The model under review builds one solid part; all positions refer to its coordinate system, in mm. A direction names the side the tool comes from. Round coordinates to 2 decimals unless told otherwise and drop trailing zeros. Loops run counter-clockwise (first coordinate to the right, second up) from the corner with the lowest first, then second, coordinate; pieces in that order, holes last. Notation, with made-up numbers: (49.25, 20.25) -> (65.25, 20.25) arc R26 ccw to (65.25, 37.25) -> close; hole circle Ø4 at (-1, -12.75). An arc over 180 degrees is marked (long way). Use a Markdown table: item, result. Add a question column.
1) For faces 5 (the flat face through (-29, 12, 0)), 6 (the flat face through (-73, -33.454, 1)), 7 (the flat face through (-65, 17.146, 1)), 8 (the flat face through (9.821, 11, 1)), 9 (the cylindrical face through (-4.345, 10.69, 0.986)), list the 3-axis set-ups (+Z, -Z, +X, -X, +Y, -Y) from which the entire face can be reached by the end or side of a thin tool; tool diameter is ignored.
2) Consider section B-B on y = 13.5. Give the boundary of the cut face in (x, z), plus the area to 3 significant figures.
3) Mouldability with a two-part tool opening along Y and no side actions: class faces 1 (the flat face through (0.818, -17.776, 0.986)), 2 (the flat face through (6.821, 16, 1)), 3 (the flat face through (2, 21.146, 1)), 4 (the flat face through (11.321, -30, 1)) as released by +Y, released by -Y, zero draft, split by the parting line, or undercut.
4) Consider section A-A on x = -11.5. Give the boundary of the cut face in (y, z).
5) Wall thickness on probe 1 along Y at (x, z) = (-65.5, 0.2); probe 2 along X at (y, z) = (15.5, 1.3); probe 3 along Y at (x, z) = (-35.5, 1.35): over which ranges is each line inside the solid? List them lowest first.
6) Insertion check: pin 1 (1 mm diameter, centred on x = 8.5, z = 1.5, fed in from -Y); pin 2 (0.8 mm diameter, centred on x = 10, z = 1, fed in from +Y); pin 3 (0.6 mm diameter, centred on y = 20, z = 1, fed in from +X). Each pin has a flat end and moves straight along its axis. Give the tip position at first contact, or say it passes through.
7) Consider section C-C on y = -3.5. Give the boundary of the cut face in (x, z), plus the area to 3 significant figures.
from build123d import *

# Parameters (mm, degrees)
EXTRUDE_1_DEPTH = 2


with BuildPart() as part:
    # 草图1 → 凸台-拉伸1 (new body)
    with BuildSketch(Plane.XY):
        Polygon((-63.278571429, -35.454285714), (-63.278571429, -33.454285714), (-65.778571429, -33.454285714), (-65.778571429, -30.954285714), (-64.278571429, -30.954285714), (-64.278571429, -28.354285714), (-65.778571429, -28.354285714), (-65.778571429, -25.354285714), (-68.778571429, -25.354285714), (-68.778571429, -28.354285714), (-70.278571429, -28.354285714), (-70.278571429, -30.954285714), (-68.778571429, -30.954285714), (-68.778571429, -33.454285714), (-77.278571429, -33.454285714), (-77.278571429, 17.145714286), (-68.778571429, 17.145714286), (-68.778571429, 14.645714286), (-70.278571429, 14.645714286), (-70.278571429, 12.045714286), (-68.778571429, 12.045714286), (-68.778571429, 9.045714286), (-65.778571429, 9.045714286), (-65.778571429, 12.045714286), (-64.278571429, 12.045714286), (-64.278571429, 14.645714286), (-65.778571429, 14.645714286), (-65.778571429, 17.145714286), (-63.278571429, 17.145714286), (-63.278571429, 21.145714286), (-59.478571429, 21.145714286), (-59.478571429, 17.145714286), (0.521428571, 17.145714286), (0.521428571, 21.145714286), (4.321428571, 21.145714286), (4.321428571, 17.145714286), (6.821428571, 17.145714286), (6.821428571, 14.645714286), (5.321428571, 14.645714286), (5.321428571, 12.045714286), (6.821428571, 12.045714286), (6.821428571, 9.045714286), (9.821428571, 9.045714286), (9.821428571, 12.045714286), (11.321428571, 12.045714286), (11.321428571, 14.645714286), (9.821428571, 14.645714286), (9.821428571, 17.145714286), (17.321428571, 17.145714286), (17.321428571, -33.454285714), (9.821428571, -33.454285714), (9.821428571, -30.954285714), (11.321428571, -30.954285714), (11.321428571, -28.354285714), (9.821428571, -28.354285714), (9.821428571, -25.354285714), (6.821428571, -25.354285714), (6.821428571, -28.354285714), (5.321428571, -28.354285714), (5.321428571, -30.954285714), (6.821428571, -30.954285714), (6.821428571, -33.454285714), (4.321428571, -33.454285714), (4.321428571, -35.454285714), (0.521428571, -35.454285714), (0.521428571, -33.454285714), (-59.478571429, -33.454285714), (-59.478571429, -35.454285714), align=None)
        with BuildLine():
            Line((-5.934446775, 11.145714286), (-52.852891654, 11.145714286))
            ThreePointArc((-52.852891654, 11.145714286), (-54.499158877, 10.653662497), (-55.605393612, 9.338917105))
            Line((-55.605393612, 9.338917105), (-62.671403465, -6.961082895))
            ThreePointArc((-62.671403465, -6.961082895), (-62.918901506, -8.154285714), (-62.671403465, -9.347488534))
            Line((-62.671403465, -9.347488534), (-55.605393612, -25.647488534))
            ThreePointArc((-55.605393612, -25.647488534), (-54.499158877, -26.962233925), (-52.852891654, -27.454285714))
            Line((-52.852891654, -27.454285714), (-5.934446775, -27.454285714))
            ThreePointArc((-5.934446775, -27.454285714), (-4.364780678, -27.010874915), (-3.259119179, -25.811717943))
            Line((-3.259119179, -25.811717943), (5.011324171, -9.511717943))
            ThreePointArc((5.011324171, -9.511717943), (5.335996575, -8.154285714), (5.011324171, -6.796853486))
            Line((5.011324171, -6.796853486), (-3.259119179, 9.503146514))
            ThreePointArc((-3.259119179, 9.503146514), (-4.364780678, 10.702303487), (-5.934446775, 11.145714286))
        make_face(mode=Mode.SUBTRACT)
    extrude(amount=EXTRUDE_1_DEPTH)


solid = part.part
Result set:
| question | item | result |
|---|---|---|
| 1 | face 5 | -Z, +X, -X, +Y, -Y |
| 1 | face 6 | +Z, -Z, -X, -Y |
| 1 | face 7 | +Z, -Z, -X, +Y |
| 1 | face 8 | +Z, -Z, +Y |
| 1 | face 9 | +Z, -Z |
| 2 | outline | (-77.28, 0) -> (-70.28, 0) -> (-70.28, 2) -> (-77.28, 2) -> close; (-64.28, 0) -> (5.32, 0) -> (5.32, 2) -> (-64.28, 2) -> close; (11.32, 0) -> (17.32, 0) -> (17.32, 2) -> (11.32, 2) -> close |
| 2 | area | 165 mm2 |
| 3 | face 1 | undercut |
| 3 | face 2 | zero draft |
| 3 | face 3 | released by +Y |
| 3 | face 4 | undercut |
| 4 | outline | (-33.45, 0) -> (-27.45, 0) -> (-27.45, 2) -> (-33.45, 2) -> close; (11.15, 0) -> (17.15, 0) -> (17.15, 2) -> (11.15, 2) -> close |
| 5 | probe 1 | -33.45 to -30.95, -28.35 to 12.05, 14.65 to 17.15 |
| 5 | probe 2 | -77.28 to -68.78, -65.78 to 6.82, 9.82 to 17.32 |
| 5 | probe 3 | -33.45 to -27.45, 11.15 to 17.15 |
| 6 | pin 1 | y = -25.35 |
| 6 | pin 2 | y = 17.15 |
| 6 | pin 3 | x = 4.32 |
| 7 | outline | (-77.28, 0) -> (-61.17, 0) -> (-61.17, 2) -> (-77.28, 2) -> close; (3.34, 0) -> (17.32, 0) -> (17.32, 2) -> (3.34, 2) -> close |
| 7 | area | 60.2 mm2 |
